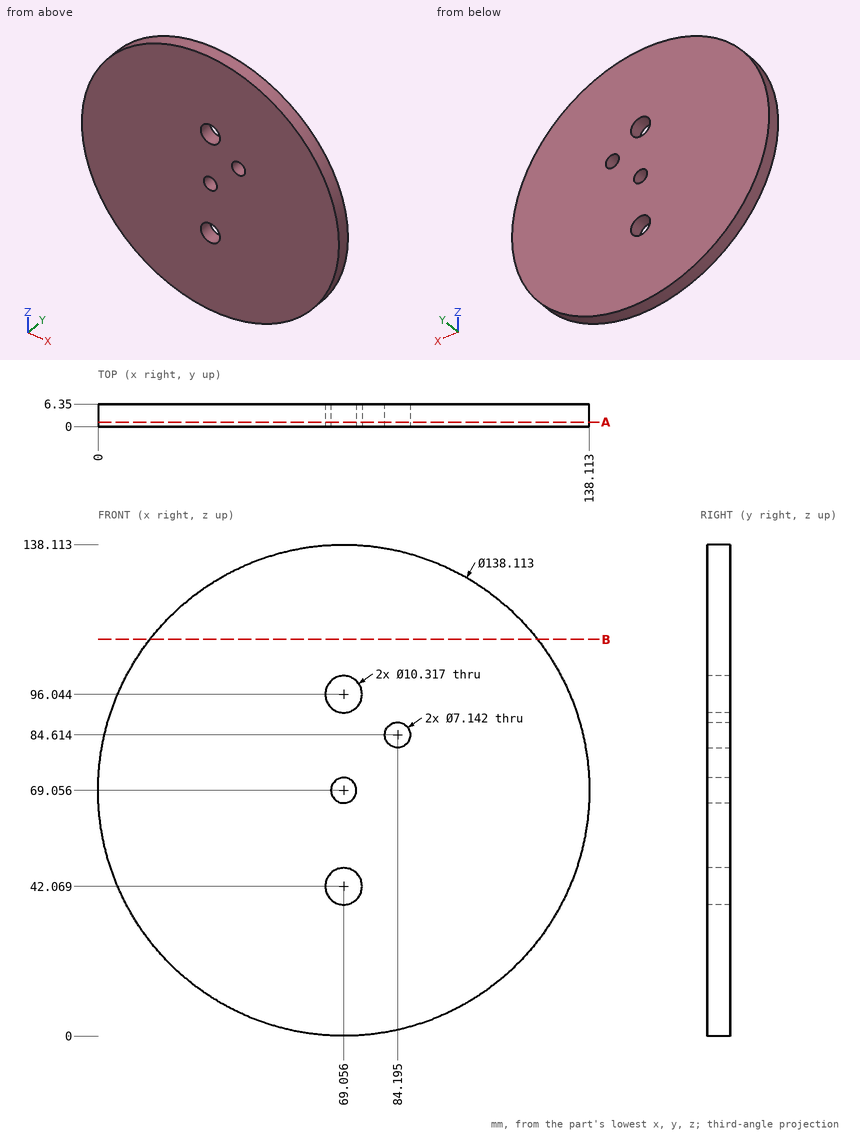
Input: dimensioned drawing with shaded views. Units: mm. Origin: part minimum x, y, z. Give positions to 0.01 mm unless a question says otherwise; leave off trailing zeros. Write each loop counter-clockwise with the first axis right and the second up, starting at its lowest first coordinate (ties: lowest second). Pieces come first, ordered by that corner, then holes.
1. Section query A-A (y = 1.25). Return the cut outline in (x, z) (1 decimal).
2. First-contact query: pin 1 (1.5 mm diameter, centred on x = 112.5, z = 44, fed in from -Y); pin 2 (1 mm diameter, centred on y = 5.5, z = 39.5, fed in from +X); pin 3 (5.5 mm diameter, centred on x = 84.19, z = 84.61, fed in from +Y); pin 4 (1.5 mm diameter, centred on x = 101, y = 4.5, fed in from -Z). Flat tips, straight axial feed; report the tip coordinate or a pass-through.
3. Material intervals for line 1 along X through (y, z) = (4.75, 70.5) (1 decimal); line 2 along Z through (x, y) = (13.5, 4) (1 decimal); line 3 along Z through (x, y) = (34, 2), sorted ascending.
4. Section query B-B (z = 111.5). Return the cut outline in (x, y).
Output values:
1. outline: circle Ø138.1 at (69.1, 69.1); hole circle Ø10.3 at (69.1, 42.1); hole circle Ø10.3 at (69.1, 96); hole circle Ø7.1 at (69.1, 69.1); hole circle Ø7.1 at (84.2, 84.6)
2. pin 1: stops at y = 0
2. pin 2: stops at x = 131.7
2. pin 3: passes through
2. pin 4: stops at z = 7.45
3. line 1: x = 0 to 65.8, 72.3 to 138.1
3. line 2: z = 28 to 110.1
3. line 3: z = 9.56 to 128.55
4. outline: (14.58, 0) - (123.53, 0) - (123.53, 6.35) - (14.58, 6.35) - close
